Source: CAD feature listing. Evaluate the final solid. Frame: model axes, mm. A direction names the side the tool comes from. Round coordinates to 2 decimals unless told otherwise and drop trailing zeros. Order: outer loops, then holes, each group sorted by start corner. A loop starts at its lowest first (then second) coordinate and runs counter-clockwise, first axis right, second up. Notation, with made-up numbers: (-35.5, 25.25) -> (-7.5, 25.25) arc R27 cw to (-7.5, 64.25) -> close; hole circle Ø10 at (3.5, 50.5). An arc over 180 degrees is marked (long way). One line per item, written item: value. Start each with the question number.
1) Mould query, pull axis X, two halves, no side actions, for faces 1 (the face through (0, -1.25, -1)), 2 (the face through (-0.867, -3.905, -0.237)), 3 (the face through (1.08, -0.63, -0.73)), 4 (the face through (2, 0, 0)). Classes: pulls with the +X half, pulls with the -X half, needs draft (parallel to the pull), parting line crosses it, or undercut.
2) Section B-B (z = -6). Return the cut outline in (x, y).
3) Pin query (flat end, axial travel): P1, Ø3, axis at y = -2, z = -10.5, coming from the +X side; P2, Ø2, axis at y = -1, z = -7, coming from the +X side; P3, Ø0.7, axis at x = -0.5, z = -0.5, coming from the +Y side. Return the tip coordinate at first contact, or that it passes through.
4) Reachability of faces 5 (the face through (0, 2, -11)), 6 (the face through (-1.088, -0.616, -0.735)), 7 (the face through (0, 0, -20)) from +Z, -Z, +X, -X, +Y, -Y: full face, straight path, thin tool, end or side. Return the list, or none.
5) Section A-A (x = 0). Return the cut outline in (y, z), and give its area (3 significant figures).
6) Ray query, L1, parallel to X at y = 1, z = -7.25; L2, parallel to Z at x = 2, y = 0.5; L3, parallel to X at y = 1.75, z = -16. Return the intervals inside material, ascending.
```python
from build123d import *

# Parameters (mm, degrees)
F2_SIZE  = 0.5
F3_R     = 4.48
F3_R_2   = 4
F4_DEPTH = 1.49


with BuildPart() as f1:
    # F0 (on Front) → F1 (revolve)
    with BuildSketch(Plane.XZ):
        Polygon((4.48, 0), (0, 0), (0, -4.48), (2, -2.48), align=None)
        Polygon((2, -2.48), (0, -4.48), (0, -20), (2, -20), align=None)
    revolve(axis=Axis((0, 0, -10), (0, 0, -1)))

    # F2
    f2_edges = [f1.edges().sort_by_distance(p)[0] for p in [
        (-2, 0, -20),
    ]]
    chamfer(f2_edges, length=F2_SIZE)

    # F3 (on Top) → F4 (cut)
    with BuildSketch(Plane.XY):
        Circle(F3_R)
        Circle(F3_R_2, mode=Mode.SUBTRACT)
        Polygon((0.7216878365, 1.25), (-0.7216878365, 1.25), (-1.443375673, 0), (-0.7216878365, -1.25), (0.7216878365, -1.25), (1.443375673, 0), align=None)
    extrude(amount=-F4_DEPTH, mode=Mode.SUBTRACT)


solid = f1.part
```
Findings:
1. face 1: undercut
1. face 2: parting line crosses it
1. face 3: undercut
1. face 4: needs draft
2. outline: circle Ø4 at (0, 0)
3. P1: x = 1.94
3. P2: x = 2
3. P3: y = 4
4. face 5: -Z
4. face 6: +Z
4. face 7: -Z, +X, -X, +Y, -Y
5. outline: (-4, -0.48) -> (-2, -2.48) -> (-2, -19.5) -> (-1.5, -20) -> (1.5, -20) -> (2, -19.5) -> (2, -2.48) -> (4, -0.48) -> (4, 0) -> (1.25, 0) -> (1.25, -1.49) -> (-1.25, -1.49) -> (-1.25, 0) -> (-4, 0) -> close
5. area: 81.9 mm2
6. L1: -1.73 to 1.73
6. L2: -2.42 to 0
6. L3: -0.97 to 0.97
